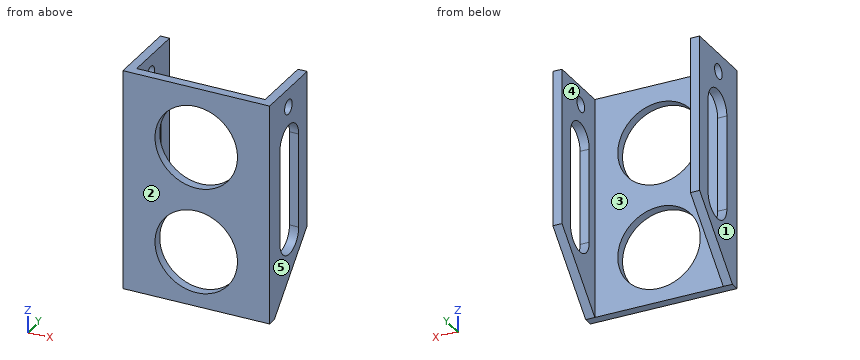
```python
from build123d import *

# Parameters (mm, degrees)
BOSS_EXTRUDE1_DEPTH     = 76.2
CUT_EXTRUDE1_REACH      = 27.4
SKETCH2_R               = 14.2875
SKETCH3_R               = 2.5527
CUT_EXTRUDE2_DEPTH      = 51.8
CUT_EXTRUDE3_DEPTH      = 48.625
CUT_EXTRUDE3_DEPTH_BACK = 4.175
CUT_EXTRUDE4_REACH      = 5.175
SKETCH5_R               = 14.2875
CUT_EXTRUDE5_DEPTH      = 48.625
CUT_EXTRUDE5_DEPTH_BACK = 4.175


with BuildPart() as part:
    # Sketch1 → Boss-Extrude1 (new body)
    with BuildSketch(Plane.XY):
        Polygon((3.175, 3.175), (3.175, 25.4), (0, 25.4), (0, 0), (50.8, 0), (50.8, 25.4), (47.625, 25.4), (47.625, 3.175), align=None)
    extrude(amount=BOSS_EXTRUDE1_DEPTH)

    # Sketch2 → Cut-Extrude1 (cut, up to next)
    with BuildSketch(Plane.XZ, mode=Mode.PRIVATE) as cut_extrude1_sk1:
        with Locations((25.4, 19.05)):
            Circle(SKETCH2_R)
    cut_extrude1_tool1 = extrude(cut_extrude1_sk1.sketch, amount=-CUT_EXTRUDE1_REACH, mode=Mode.PRIVATE) & part.part
    add(cut_extrude1_tool1.solids().sort_by_distance((25.4, 0, 19.05))[0], mode=Mode.SUBTRACT)

    # Sketch3 → Cut-Extrude2 (cut, through all)
    with BuildSketch(Plane.ZY):
        with Locations((69.85, 12.7)):
            Circle(SKETCH3_R)
    extrude(amount=-CUT_EXTRUDE2_DEPTH, mode=Mode.SUBTRACT)

    # Sketch4 → Cut-Extrude3 (cut, two sides)
    with BuildSketch(Plane.ZY.offset(-47.625)) as cut_extrude3_sk:
        Polygon((0, 3.175), (22.225, 25.4), (0, 25.4), align=None)
    extrude(amount=CUT_EXTRUDE3_DEPTH, mode=Mode.SUBTRACT)
    extrude(cut_extrude3_sk.sketch, amount=-CUT_EXTRUDE3_DEPTH_BACK, mode=Mode.SUBTRACT)

    # Sketch5 → Cut-Extrude4 (cut, up to next)
    with BuildSketch(Plane(origin=(0, 3.175, 0), x_dir=(1, 0, 0), z_dir=(0, 1, 0)), mode=Mode.PRIVATE) as cut_extrude4_sk1:
        with Locations((25.4, -55.5625)):
            Circle(SKETCH5_R)
    cut_extrude4_tool1 = extrude(cut_extrude4_sk1.sketch, amount=-CUT_EXTRUDE4_REACH, mode=Mode.PRIVATE) & part.part
    add(cut_extrude4_tool1.solids().sort_by_distance((25.4, 3.175, 55.5625))[0], mode=Mode.SUBTRACT)

    # Sketch6 → Cut-Extrude5 (cut, two sides)
    with BuildSketch(Plane.ZY.offset(-47.625)) as cut_extrude5_sk:
        with BuildLine():
            Line((24.485892943, 19.673757433), (57.04010233, 19.673757433))
            ThreePointArc((57.04010233, 19.673757433), (63.39010233, 13.323757433), (57.04010233, 6.973757433))
            Line((57.04010233, 6.973757433), (24.485892943, 6.973757433))
            ThreePointArc((24.485892943, 6.973757433), (18.135892943, 13.323757433), (24.485892943, 19.673757433))
        make_face()
    extrude(amount=CUT_EXTRUDE5_DEPTH, mode=Mode.SUBTRACT)
    extrude(cut_extrude5_sk.sketch, amount=-CUT_EXTRUDE5_DEPTH_BACK, mode=Mode.SUBTRACT)


solid = part.part
```
Geometry check sheet. Reference: the model listing, model coordinates, mm. Face numbers are marked on the shaded views. A direction names the side the tool comes from. Round coordinates to 2 decimals unless told otherwise and drop trailing zeros. Order: outer loops, then holes, each group sorted by start corner. A loop starts at its lowest first (then second) coordinate and runs counter-clockwise, first axis right, second up. Notation, with made-up numbers: (-26.75, 4) -> (-3.75, 4) arc R11 cw to (-3.75, 25) -> close; hole circle Ø11 at (67.25, -19). An arc over 180 degrees is marked (long way). Return JSON: item names as keys, results as strings. Group by question number.
Q1. Section check B-B, the plane z = 59. Record the boundary of the cut face in (x, y) (3 decimals), plus the area to 3 significant figures.
Q2. Gauge pin test, flat end, axial feed: pin 1 (8 mm diameter, centred on x = 38, z = 17, fed in from +Y) (3 decimals). Record the tip position at first contact, or that the pin passes through.
Q3. Section check C-C, the plane y = 7.75. Record the boundary of the cut face in (x, z) (3 decimals).
Q4. Section check D-D, the plane y = 22.25. Record the boundary of the cut face in (x, z) (3 decimals), plus the area to 3 significant figures.
Q5. Release check for a two-part mould opening along X. For the marked faces 1, 2 and 3 record: released by +X, released by -X, zero draft, split by the parting line, or undercut.
Q6. Material ranges on probe 1 along X at (y, z) = (15.25, 67) (3 decimals); probe 2 along Y at (x, z) = (49.15, 69.85); probe 3 along Y at (x, z) = (46.5, 65) (3 decimals), recorded low to high. Write a range as from..to.
Q7. Tool access check on the marked faces 4 and 5. Record the directions out of +Z, -Z, +X, -X, +Y, -Y that give a thin tool (end or side, any length) a straight path to the whole face; none if there is none.
Q8. Section check A-A, the plane x = 25.4. Count the separate pieces of the cut face and the enclosed holes in it, plus the area to 3 significant figures.
Numbers:
{
 "1": {"outline": "(0, 0) -> (11.532, 0) -> (11.532, 3.175) -> (3.175, 3.175) -> (3.175, 7.284) -> (0, 7.284) -> close; (0, 19.364) -> (3.175, 19.364) -> (3.175, 25.4) -> (0, 25.4) -> close; (39.268, 0) -> (50.8, 0) -> (50.8, 7.284) -> (47.625, 7.284) -> (47.625, 3.175) -> (39.268, 3.175) -> close; (47.625, 19.364) -> (50.8, 19.364) -> (50.8, 25.4) -> (47.625, 25.4) -> close", "area": "138 mm^2"},
 "2": {"pin 1": "y = 3.175"},
 "3": {"outline": "(0, 4.575) -> (3.175, 4.575) -> (3.175, 21.444) -> (0, 21.444) -> close; (0, 60.082) -> (3.175, 60.082) -> (3.175, 76.2) -> (0, 76.2) -> close; (47.625, 4.575) -> (50.8, 4.575) -> (50.8, 21.444) -> (47.625, 21.444) -> close; (47.625, 60.082) -> (50.8, 60.082) -> (50.8, 76.2) -> (47.625, 76.2) -> close"},
 "4": {"outline": "(0, 19.075) -> (3.175, 19.075) -> (3.175, 76.2) -> (0, 76.2) -> close; (47.625, 19.075) -> (50.8, 19.075) -> (50.8, 76.2) -> (47.625, 76.2) -> close", "area": "363 mm^2"},
 "5": {"face 1": "released by -X", "face 2": "zero draft", "face 3": "undercut"},
 "6": {"probe 1": "0..3.175, 47.625..50.8", "probe 2": "0..10.15, 15.25..25.4", "probe 3": "0..3.175"},
 "7": {"face 4": "+Z, -Z, +Y", "face 5": "+Z, -Z, +X, +Y, -Y"},
 "8": {"separate pieces": "3", "enclosed holes": "0", "area": "60.5 mm^2"}
}
